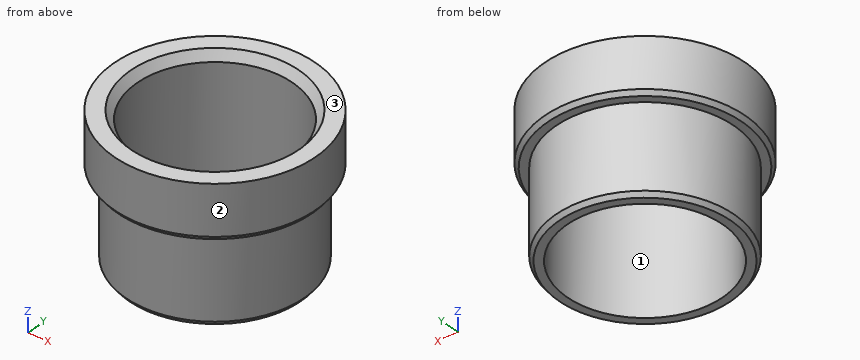
```python
from build123d import *
from OCP.BRepFilletAPI import BRepFilletAPI_MakeChamfer

# Parameters (mm, degrees)
CHAMFER2_SIZE  = 0.5334
CHAMFER2_SIZE2 = 0.40194573


with BuildPart() as part:
    # Sketch2 → Revolve1 (revolve)
    with BuildSketch(Plane(origin=(0, 0, 0), x_dir=(0, 0, -1), z_dir=(1, 0, 0)), mode=Mode.PRIVATE) as revolve1_sk:
        Polygon((8.636, 9.525), (8.636, 10.922), (-2.032, 10.922), (-2.032, 12.319), (-8.636, 12.319), (-8.636, 10.328891461), (-7.5692, 9.525), align=None)
    revolve(revolve1_sk.sketch.rotate(Axis((0, 0, -8.636), (0, 0, 1)), 90), axis=Axis((0, 0, -8.636), (0, 0, 1)))

    # Chamfer2: one chamfer whose edges measure the first distance from different faces: ONE call of the kernel's chamfer builder (chamfer() names one face for all edges)
    chamfer2_edges_1 = [part.edges().sort_by_distance(p)[0] for p in [
        (12.319, 0, 2.032),
    ]]
    chamfer2_side_1 = [part.faces().sort_by_distance(p)[0] for p in [
        (12.319, 0, 5.334),
    ]]
    chamfer2_edges_2 = [part.edges().sort_by_distance(p)[0] for p in [
        (10.922, 0, -8.636),
    ]]
    chamfer2_side_2 = [part.faces().sort_by_distance(p)[0] for p in [
        (10.922, 0, -3.302),
    ]]
    chamfer2 = BRepFilletAPI_MakeChamfer(part.part.solid().wrapped)
    for e in chamfer2_edges_1:
        chamfer2.Add(CHAMFER2_SIZE, CHAMFER2_SIZE2, e.wrapped, chamfer2_side_1[0].wrapped)  # the first distance lies on this face
    for e in chamfer2_edges_2:
        chamfer2.Add(CHAMFER2_SIZE, CHAMFER2_SIZE2, e.wrapped, chamfer2_side_2[0].wrapped)  # the first distance lies on this face
    add(Compound.cast(chamfer2.Shape()), mode=Mode.REPLACE)


solid = part.part
```
Input: part model. Units: mm. Frame: model coordinates. Face numbers are marked on the shaded views. Coordinates: 2 decimals unless noted, no trailing zeros. Loops run counter-clockwise (first coordinate to the right, second up) from the corner with the lowest first, then second, coordinate; pieces in that order, holes last.
Q1. Section D-D, the plane z = -0.5. Return the cut outline in (x, y) (3 decimals).
Results are:
outline: circle Ø21.844 at (0, 0); hole circle Ø19.05 at (0, 0)
Q2. Contact query for flat-ended pins moving along their axis: pin 1 (6 mm diameter, centred on x = 7.5, z = -6.5, fed in from -Y); pin 2 (1 mm diameter, centred on x = 3, z = -1.5, fed in from +Y); pin 3 (4 mm diameter, centred on y = -9.5, z = 3, fed in from +X). Output: stop coordinate, or through.
Results are:
pin 1: stops at y = -9.95
pin 2: stops at y = 10.63
pin 3: stops at x = 9.77
Q3. Mould query, pull axis X, two halves, no side actions, for the marked faces 1, 2 and 3. Classes: +X half, -X half, draft (parallel to the pull), parting line (faces both ways), or undercut.
Results are:
face 1: undercut
face 2: parting line
face 3: draft
Q4. Section C-C, the plane z = 6.5. Return the cut outline in (x, y) (3 decimals), and give its area (3 significant figures).
Results are:
outline: circle Ø24.638 at (0, 0); hole circle Ø19.05 at (0, 0)
area: 192 mm2
Q5. Line query: line 1 along Y through (x, z) = (0, -5) (3 decimals); line 2 along Z through (x, y) = (0.75, -11.5); line 3 along Y through (x, z) = (-0.5, 5.25). Output: solid intervals per line, ascending.
Results are:
line 1: y = -10.922 to -9.525, 9.525 to 10.922
line 2: z = 2.03 to 8.64
line 3: y = -12.31 to -9.51, 9.51 to 12.31
Q6. Section A-A, the plane y = 0. Return the cut outline in (x, z) (3 decimals).
Results are:
outline: (-12.319, 2.565) - (-11.917, 2.032) - (-10.922, 2.032) - (-10.922, -8.103) - (-10.52, -8.636) - (-9.525, -8.636) - (-9.525, 7.569) - (-10.329, 8.636) - (-12.319, 8.636) - close; (9.525, -8.636) - (10.52, -8.636) - (10.922, -8.103) - (10.922, 2.032) - (11.917, 2.032) - (12.319, 2.565) - (12.319, 8.636) - (10.329, 8.636) - (9.525, 7.569) - close
